Can you work these out from the drawing? Everything is in mm from the part's minimum corner. A direction names the side the tool comes from. Coordinates: 2 decimals unless noted, no trailing zeros. Loops run counter-clockwise (first coordinate to the right, second up) from the corner with the lowest first, then second, coordinate; pieces in that order, holes last.
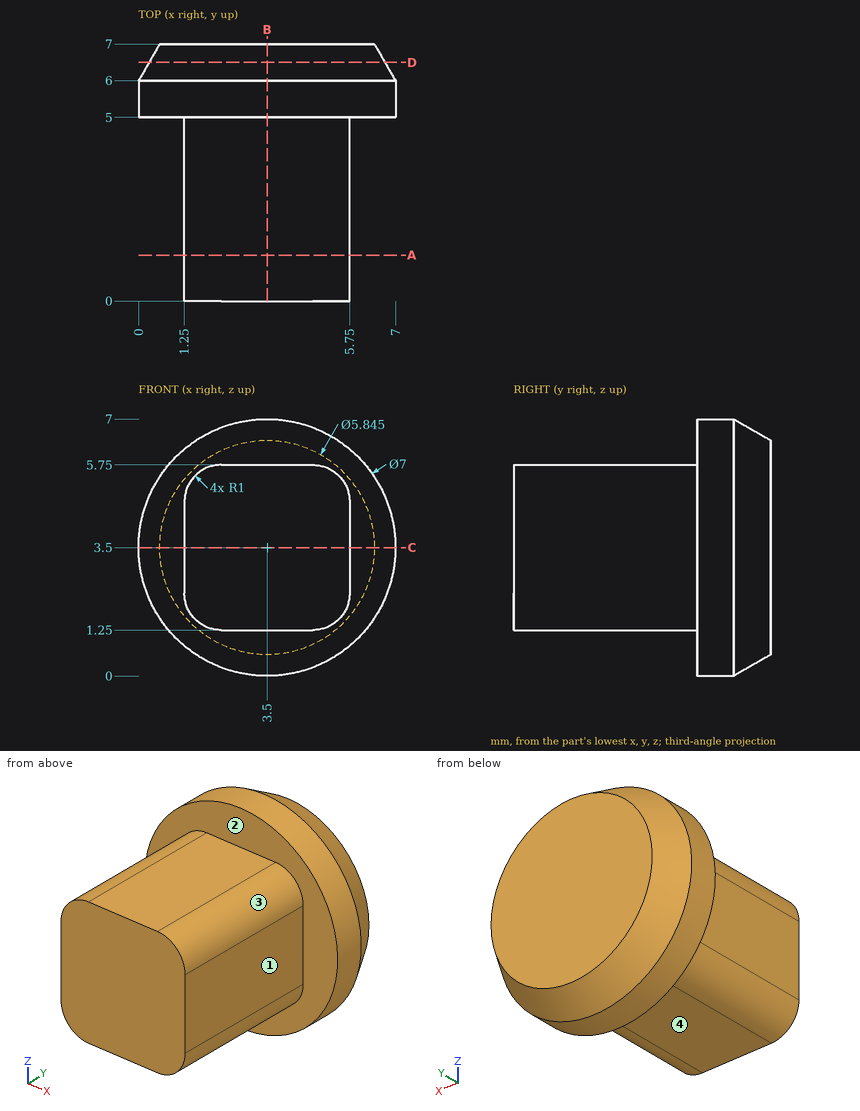
1. I want a section at D-D (y = 6.5). Please give me the cut outline in (x, z).
2. I want a section at C-C (z = 3.5). Please give me the cut outline in (x, y).
3. I want a section at A-A (y = 1.25). Please give me the cut outline in (x, z), then the cut area to 3 significant figures.
4. On a 3-axis mill with a long thin cutter (end or side, diameter ignored), from which of +Z, -Z, +X, -X, +Y, -Y can I reach the whole of each face in a straight line? I mean the marked faces 1, 2, 3 and 4. Say none if no direction works.
5. I need wall thicknesses on line 1 along X through (y, z) = (1, 4.25); line 2 along Y through (x, z) = (3.75, 6). Which ranges of each line are inside material? Lowest first, please.
6. For pin 1 (0.8 mm diameter, centred on x = 3.5, y = 3, fed in from -Z); pin 2 (2 mm diameter, centred on x = 1.5, z = 4.5, fed in from -Y); pin 3 (2 mm diameter, centred on y = 3.5, z = 2, fed in from -X); pin 4 (2 mm diameter, centred on y = 3, z = 3.5, fed in from +X), each with a flat end and sliding along its axis, tell me the tip position at first contact or that it passes through.
7. I want a section at B-B (x = 3.5). Please give me the cut outline in (y, z).
Response values:
1. outline: circle Ø6.42 at (3.5, 3.5)
2. outline: (0, 5) - (1.25, 5) - (1.25, 0) - (5.75, 0) - (5.75, 5) - (7, 5) - (7, 6) - (6.42, 7) - (0.58, 7) - (0, 6) - close
3. outline: (1.25, 2.25) arc R1 ccw to (2.25, 1.25) - (4.75, 1.25) arc R1 ccw to (5.75, 2.25) - (5.75, 4.75) arc R1 ccw to (4.75, 5.75) - (2.25, 5.75) arc R1 ccw to (1.25, 4.75) - close
3. area: 19.4 mm2
4. face 1: +Z, -Z, +X, -Y
4. face 2: -Y
4. face 3: +Z, +X, -Y
4. face 4: -Z, +X, -X, -Y
5. line 1: x = 1.25 to 5.75
5. line 2: y = 5 to 7
6. pin 1: stops at z = 1.25
6. pin 2: stops at y = 0
6. pin 3: stops at x = 1.25
6. pin 4: stops at x = 5.75
7. outline: (0, 1.25) - (5, 1.25) - (5, 0) - (6, 0) - (7, 0.58) - (7, 6.42) - (6, 7) - (5, 7) - (5, 5.75) - (0, 5.75) - close
